Check sheet for the drawn part. Datum: minimum x, y, z corner. Units: mm. A direction names the side the tool comes from. Coordinates: 2 decimals unless noted, no trailing zeros. Write each loop counter-clockwise with the first axis right and the second up, starting at its lowest first coordinate (ties: lowest second). Pieces come first, ordered by that corner, then holes. Notation, with made-up numbers: (29, -14) -> (35, -14) arc R9 ccw to (35, -8) -> close; hole circle Ø5 at (33, 41). An arc over 180 degrees is marked (long way). Answer in a Markdown table with one row per item.
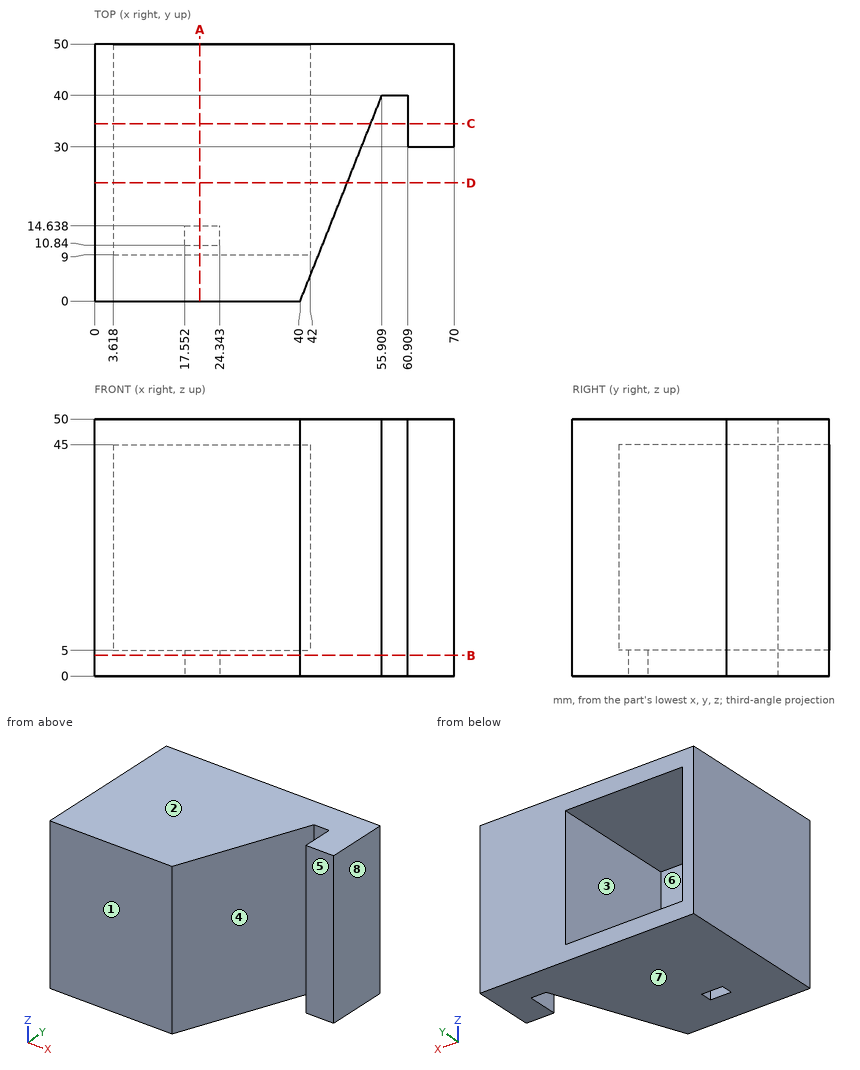
1. Sectioned sample at A-A, the plane x = 20.5. Record the cut outline in (y, z).
Findings below:
| item | result |
|---|---|
| outline | (0, 0) -> (10.84, 0) -> (10.84, 5) -> (9, 5) -> (9, 45) -> (50, 45) -> (50, 50) -> (0, 50) -> close; (14.64, 0) -> (50, 0) -> (50, 5) -> (14.64, 5) -> close |
2. Sectioned sample at C-C, the plane y = 34.5. Record the cut outline in (x, z), and give its area (3 significant figures).
Findings below:
| item | result |
|---|---|
| outline | (0, 0) -> (53.72, 0) -> (53.72, 50) -> (0, 50) -> close; (60.91, 0) -> (70, 0) -> (70, 50) -> (60.91, 50) -> close; hole (3.62, 5) -> (42, 5) -> (42, 45) -> (3.62, 45) -> close |
| area | 1,610 mm² |
3. Go/stop test with flat-tipped pins: pin 1 (3 mm diameter, centred on y = 13, z = 3.5, fed in from +X); pin 2 (11.5 mm diameter, centred on x = 29, z = 32.5, fed in from +Y); pin 3 (7.5 mm diameter, centred on x = 67, z = 13.5, fed in from -Y). Record where each tip stops, or that it passes through.
Findings below:
| item | result |
|---|---|
| pin 1 | stops at x = 45.77 |
| pin 2 | stops at y = 9 |
| pin 3 | stops at y = 30 |
4. Release check for a two-part mould opening along Z. For the marked faces 1, 2 and 3 record: released by +Z, released by -Z, zero draft, split by the parting line, or undercut.
Findings below:
| item | result |
|---|---|
| face 1 | zero draft |
| face 2 | released by +Z |
| face 3 | undercut |
5. Access from +Z, -Z, +X, -X, +Y, -Y to the whole of each face (thin tool, end or side, straight path). Record for the marked faces 4, 5, 6, 7 and 8.
Findings below:
| item | result |
|---|---|
| face 4 | +Z, -Z, -Y |
| face 5 | +Z, -Z, +X, -Y |
| face 6 | +Y |
| face 7 | -Z, +X, -X, +Y, -Y |
| face 8 | +Z, -Z, +X, +Y, -Y |
6. Material ranges on probe 1 along Z at (x, y) = (25.5, 22); probe 2 along Y at (x, z) = (14, 26.5); probe 3 along X at (y, z) = (23.5, 29), recorded low to high. Write a range as from..to.
Findings below:
| item | result |
|---|---|
| probe 1 | z = 0..5, 45..50 |
| probe 2 | y = 0..9 |
| probe 3 | x = 0..3.62, 42..49.35 |
7. Sectioned sample at B-B, the plane z = 4. Record the cut outline in (x, y).
Findings below:
| item | result |
|---|---|
| outline | (0, 0) -> (40, 0) -> (55.91, 40) -> (60.91, 40) -> (60.91, 30) -> (70, 30) -> (70, 50) -> (0, 50) -> close; hole (17.55, 10.84) -> (24.34, 10.84) -> (24.34, 14.64) -> (17.55, 14.64) -> close |
8. Sectioned sample at D-D, the plane y = 23. Record the cut outline in (x, z).
Findings below:
| item | result |
|---|---|
| outline | (0, 0) -> (49.15, 0) -> (49.15, 50) -> (0, 50) -> close; hole (3.62, 5) -> (42, 5) -> (42, 45) -> (3.62, 45) -> close |
